Autodesk Inventor part; units mm, degrees
ref_plane "Work Plane1" through (7.5584, 0, 0) normal (0, 0, -1) x (1, 0, 0)
ref_plane "YZ Plane" through (0, 0, 0) normal (1, 0, 0) x (0, 1, 0)
ref_plane "XZ Plane" through (0, 0, 0) normal (0, 1, 0) x (-1, 0, 0)
sketch "Sketch1" plane through (0, 0, 0) normal (0, 0, 1) x (1, 0, 0)
  line L0 (-12.7, 0) -> (76.2, 0)
  line L1 (0, 0) -> (63.5, 0)
  line L2 (63.5, 0) -> (63.5, 4.7625)
  line L3 (63.5, 4.7625) -> (38.1, 4.7625)
  line L4 (38.1, 4.7625) -> (36.5125, 4.7625)
  line L5 (36.5125, 4.7625) -> (5.842, 4.7625)
  line L6 (5.842, 4.7625) -> (5.842, 4.7625)
  line L7 (5.842, 4.7625) -> (1.313, 8.6995)
  line L8 (1.313, 8.6995) -> (0, 8.6995)
  line L9 (0, 8.6995) -> (0, 0)
  line L10 (0, -1.7399) -> (0, 10.4394)
  line L11 (38.1, 4.7625) -> (5.842, 4.7625) construction
  dimension "d2" = 63.5
  dimension "d3" = 5.842
  dimension "d4" = 25.4
  dimension "d5" = 1.5875
  dimension "d6" = 9.525
  dimension "d7" = 9.525
  dimension "d8" = 9.525
  dimension "d9" = 17.399
  dimension "d10" = 41
revolve "Body" add sketch "Sketch1" angle 360 about axis through (0, 0, 0) along (1, 0, 0)
sketch "Sketch2" plane through (0, 0, 0) normal (-1, 0, 0) x (0, 0, 1)
  circle A0 centre (0, 0) radius 8.6995
  line L0 (-12.1793, 0) -> (12.1793, 0)
  line L1 (-8.6995, 0) -> (-8.6995, 1.1938)
  line L2 (-8.6995, 1.1938) -> (8.6995, 1.1938)
  line L3 (8.6995, 0) -> (8.6995, 1.1938)
  line L4 (-8.6995, 0) -> (-8.6995, -1.1938)
  line L5 (-8.6995, -1.1938) -> (8.6995, -1.1938)
  line L6 (8.6995, 0) -> (8.6995, -1.1938)
  dimension "d15" = 2.3876
extrude "Slot" cut sketch "Sketch2" against normal blind 2.6924 contours L0 A0 L2 | L6 L5 A0 | A0 L5 L0 | A0 L2 L3 | L1 L2 A0 | A0 L5 L4
thread "Thread"
ref_plane "Work Plane1" through (7.5584, 0, 0) normal (0, 0, -1) x (1, 0, 0)
equation "\"d2\" = NLG"
equation "\"d3\" = KOH"
equation "\"d4\" = GEL"
equation "\"d5\" = GAL"
equation "\"d6\" = GD"
equation "\"d7\" = BDM"
equation "\"d8\" = KOD1"
equation "\"d9\" = KOD"
equation "\"d10\" = 0.5 * SEWI"
equation "\"d15\" = SBR"
equation "\"d16\" = STI"
equation "\"d12\" = GEL"
equation "\"NND\" = 9.525"
equation "\"NLG\" = 63.5"
equation "\"GEL\" = 25.4"
equation "\"KOH\" = 5.842"
equation "\"KOD\" = 17.399"
equation "\"SBR\" = 2.3876"
equation "\"STI\" = 2.6924"
equation "\"GAL\" = 1.5875"
equation "\"SPD\" = 7.14375"
equation "\"GD\" = NND"
equation "\"KOD1\" = NND"
equation "\"BDM\" = NND"
equation "\"SEWI\" = 82deg"
equation "\"GUL\" = 0.0254"
equation "\"THREADDIA\" = 9.525"
equation "\"TOA\" = 30deg"
equation "\"GD1\" = SPD"
properties part number "ANSI B18.6.3 - 3/8-16 x 2 1/2, SFCHMSI(1)" material "Steel, Mild"
Source: CAD feature listing. Evaluate the final solid. Frame: model axes, mm. A direction names the side the tool comes from. Give positions to 0.01 mm unless a question says otherwise; leave off trailing zeros. Loops run counter-clockwise (first coordinate to the right, second up) from the corner with the lowest first, then second, coordinate; pieces in that order, holes last. Notation, with made-up numbers: (34, -19) -> (64, -19) arc R28 ccw to (64, 14) -> close; hole circle Ø1 at (87.25, 16.25). An arc over 180 degrees is marked (long way). Use a Markdown table: item, result. Add a question column.
(1) Access query for faces 1 (the face through (0.647, -8.698, -0.175)), 2 (the face through (1, -1.194, 0)), 3 (the face through (34.27, -3.78, 2.9)). Directions: +Z, -Z, +X, -X, +Y, -Y. A direction counts if a zero-diameter tool reaches every point of the face in a straight line with its end or side. Return the directions, or none.
(2) Section query C-C (x = 32.5). Output: boundary loops of the cut face in (y, z) (1 decimal), then the cut area to 3 significant figures.
(3) Ray query, line 1 (Y direction, x = 26.5, z = -0.25); line 2 (Y direction, x = 28, z = 3); line 3 (X direction, y = -2, z = 4.5). Return the intervals inside material, ascending.
(4) Section query A-A (y = 0). Output: boundary loops of the cut face in (x, z), then the cut area to 3 significant figures.
(5) Section query B-B (z = 0). Output: boundary loops of the cut face in (x, y), then the cut area to 3 significant figures.
(6) First-contact query: pin 1 Ø8 at (x, z) = (15.5, 0.5) entering from -Y; pin 2 Ø10 at (x, y) = (54, 2.5) entering from +Z; pin 3 Ø2 at (x, y) = (19, 1) entering from -Z. Flat tips, straight axial feed; report the tip coordinate or a pass-through.
Checked values:
| question | item | result |
|---|---|---|
| 1 | face 1 | +X, -X, -Y |
| 1 | face 2 | +Z, -Z, -X |
| 1 | face 3 | +X |
| 2 | outline | circle Ø9.5 at (0, 0) |
| 2 | area | 71.3 mm^2 |
| 3 | line 1 | -4.76 to 4.76 |
| 3 | line 2 | -3.7 to 3.7 |
| 3 | line 3 | 0 to 5.66 |
| 4 | outline | (2.69, -7.5) -> (5.84, -4.76) -> (63.5, -4.76) -> (63.5, 4.76) -> (5.84, 4.76) -> (2.69, 7.5) -> close |
| 4 | area | 588 mm^2 |
| 5 | outline | (0, -8.7) -> (1.31, -8.7) -> (5.84, -4.76) -> (63.5, -4.76) -> (63.5, 4.76) -> (5.84, 4.76) -> (1.31, 8.7) -> (0, 8.7) -> (0, 1.19) -> (2.69, 1.19) -> (2.69, -1.19) -> (0, -1.19) -> close |
| 5 | area | 627 mm^2 |
| 6 | pin 1 | y = -4.76 |
| 6 | pin 2 | z = 4.76 |
| 6 | pin 3 | z = -4.76 |
